Could you check a few things on this model? Use its own coordinates, in mm. Face numbers are marked on the shaded views. Coordinates: 2 decimals unless noted, no trailing zeros. Write each loop counter-clockwise with the first axis right and the second up, starting at its lowest first coordinate (ties: lowest second). Pieces come first, ordered by that corner, then holes.
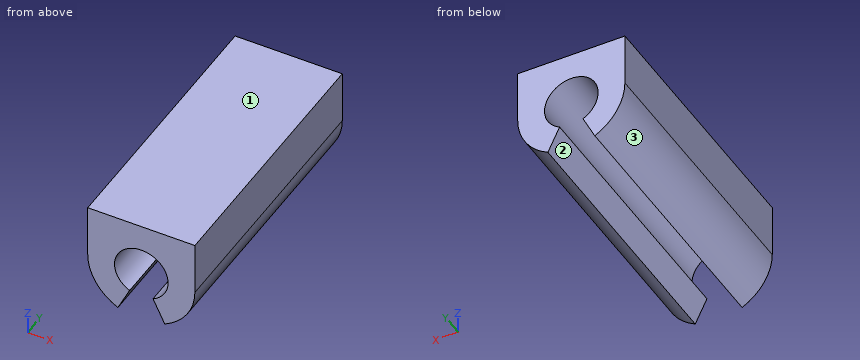
```python
from build123d import *

# Parameters (mm, degrees)
F0_R     = 1
F1_DEPTH = 5
F3_DEPTH = 10.001


# Not quite as in the source:
# - a feature of the source that left no trace in its solid (it failed there, or was rolled back) is left out


with BuildPart() as f1:
    # F0 (on Front) → F1 (new body, symmetric)
    with BuildSketch(Plane.XZ):
        with BuildLine():
            Line((-2, 2), (-2, 0))
            ThreePointArc((-2, 0), (0, -2), (2, 0))
            Line((2, 0), (2, 2))
            Line((2, 2), (0, 2))
            Line((0, 2), (-2, 2))
        make_face()
        Circle(F0_R, mode=Mode.SUBTRACT)
    extrude(amount=F1_DEPTH, both=True)

    # F2 (on face) → F3 (cut, through all)
    with BuildSketch(Plane.XZ.offset(5)):
        with BuildLine():
            Line((0.875, -1.7984368212), (0, 0))
            Line((0, 0), (-0.875, -1.7984368212))
            ThreePointArc((-0.875, -1.7984368212), (0, -2), (0.875, -1.7984368212))
        make_face()
    extrude(amount=-F3_DEPTH, mode=Mode.SUBTRACT)


solid = f1.part
```
1. I want a section at D-D on x = -1.6. Please give me the cut outline in (y, z), plus the area to 3 significant figures.
Verdict:
outline: (-5, -1.2) - (5, -1.2) - (5, 2) - (-5, 2) - close
area: 32.0 mm2
2. I want a section at B-B on y = 4. Please give me the cut outline in (x, z) (1 decimal).
Verdict:
outline: (-2, 0) arc R2 ccw to (-0.9, -1.8) - (-0.4, -0.9) arc R1 cw (long way) to (0.4, -0.9) - (0.9, -1.8) arc R2 ccw to (2, 0) - (2, 2) - (-2, 2) - close
3. If we mould it in two halves opening along X, with no side actions, what happens to the marked faces 1, 2 and 3? For each: pulls with the +X half, pulls with the -X half, needs draft (parallel to the pull), parting line crosses it, or undercut.
Verdict:
face 1: needs draft
face 2: undercut
face 3: pulls with the -X half
4. Please list where these lines run through material, in increasing order: line 1 along X through (y, z) = (0.25, 0); line 2 along X through (y, z) = (4, -1.2); line 3 along Z through (x, y) = (-0.6, 1.25).
Verdict:
line 1: x = -2 to -1, 1 to 2
line 2: x = -1.6 to -0.58, 0.58 to 1.6
line 3: z = -1.23 to -0.8, 0.8 to 2
5. I want a section at C-C on z = -1. Please give me the cut outline in (x, y).
Verdict:
outline: (-1.73, -5) - (-0.49, -5) - (-0.49, 5) - (-1.73, 5) - close; (0.49, -5) - (1.73, -5) - (1.73, 5) - (0.49, 5) - close
6. For pin 1 (1 mm diameter, centred on x = 0, y = 0, fed in from -Z), with a flat end and sliding along its axis, tell me the tip position at first contact or that it passes through.
Verdict:
pin 1: stops at z = -1.03
7. I want a section at A-A on x = -0.65. Please give me the cut outline in (y, z), plus the area to 3 significant figures.
Verdict:
outline: (-5, -1.34) - (5, -1.34) - (5, -0.76) - (-5, -0.76) - close; (-5, 0.76) - (5, 0.76) - (5, 2) - (-5, 2) - close
area: 18.2 mm2
